Model file for the job. Use its own axes, mm. A direction names the side the tool comes from. Round coordinates to 2 decimals unless told otherwise and drop trailing zeros. Loops run counter-clockwise (first coordinate to the right, second up) from the corner with the lowest first, then second, coordinate; pieces in that order, holes last. Notation, with made-up numbers: (49.25, 85) - (64.25, 85) arc R16 cw to (64.25, 101) - close; hole circle Ø9 at (86, 0.5). An arc over 180 degrees is marked (long way). Use one line per item in the form item = value.
from build123d import *

# Parameters (mm, degrees)
F0_W     = 2032
F0_H     = 508
F1_DEPTH = 762
F2_W     = 591.2553668022
F2_H     = 534.2325568199
F3_DEPTH = 2032


with BuildPart() as f1:
    # F0 (on Front) → F1 (new body)
    with BuildSketch(Plane.XZ):
        Polygon((1016, 0), (0, 0), (-1016, 0), (-1016, -76.2), (1016, -76.2), align=None)
        Polygon((-1016, 0), (0, 0), (1016, 0), (1016, 508), (-1016, 508), align=None)
        with Locations((0, 762)):
            Rectangle(F0_W, F0_H)
        Polygon((-669.1186458851, 1351.5236000156), (-1016, 1016), (1016, 1016), (680.4763999844, 1362.8813541149), align=None)
    extrude(amount=F1_DEPTH)

    # F2 (on face) → F3 (cut)
    with BuildSketch(Plane(origin=(-1016, 0, 0), x_dir=(0, -1, 0), z_dir=(-1, 0, 0))):
        with Locations((401.707559824, 237.3584806919)):
            Rectangle(F2_W, F2_H)
    extrude(amount=-F3_DEPTH, mode=Mode.SUBTRACT)


solid = f1.part
1. Tool access for faces 1 (the flat face through (-14, -106.08, 234)), 2 (the flat face through (-1016, -376, 720)): list every direction of +Z, -Z, +X, -X, +Y, -Y with a clear straight run to the whole face (end or side of a thin tool).
Geometry check:
face_1 = +X, -X
face_2 = +Z, -Z, -X, +Y, -Y
2. Cut at B-B, the plane y = -425. Give the cut face in (x, z).
Geometry check:
outline = (-1016, -76.2) - (1016, -76.2) - (1016, -29.76) - (-1016, -29.76) - close; (-1016, 504.47) - (1016, 504.47) - (1016, 1016) - (680.48, 1362.88) - (-669.12, 1351.52) - (-1016, 1016) - close
3. Pull direction Z, two halves, no side cores. Call faces 3 (the flat face through (-14, -376, -76.2)), 4 (the flat face through (-14, -697.335, 234)), 5 (the flat face through (1016, -376, 705)), 6 (the flat face through (-14, -398, -29.758)): +Z half, -Z half, draft (parallel to the pull), parting line (faces both ways), or undercut.
Geometry check:
face_3 = -Z half
face_4 = undercut
face_5 = draft
face_6 = undercut
4. Wall check: probe 1 along Y at (x, z) = (304, 341.5); probe 2 along Z at (x, y) = (644, -176); probe 3 along Z at (x, y) = (-57.5, -514). Give the ranges that are in metal, low to high.
Geometry check:
probe_1 = -762 to -697.34, -106.08 to 0
probe_2 = -76.2 to -29.76, 504.47 to 1362.57
probe_3 = -76.2 to -29.76, 504.47 to 1356.67
5. Cut at D-D, the plane y = -69. Give the cut face in (x, z).
Geometry check:
outline = (-1016, -76.2) - (1016, -76.2) - (1016, 1016) - (680.48, 1362.88) - (-669.12, 1351.52) - (-1016, 1016) - close
6. Cut at A-A, the plane z = 233. Give the cut face in (x, y), plus the area to 3 significant figures.
Geometry check:
outline = (-1016, -762) - (1016, -762) - (1016, -697.34) - (-1016, -697.34) - close; (-1016, -106.08) - (1016, -106.08) - (1016, 0) - (-1016, 0) - close
area = 347,000 mm^2
7. Cut at C-C, the plane x = 724.5. Give the cut face in (y, z), plus the area to 3 significant figures.
Geometry check:
outline = (-762, -76.2) - (0, -76.2) - (0, 1317.37) - (-762, 1317.37) - close; hole (-697.34, -29.76) - (-106.08, -29.76) - (-106.08, 504.47) - (-697.34, 504.47) - close
area = 746,000 mm^2
8. Flat gauge pins, fed straight in: pin 1 (1 mm diameter, centred on x = -770, y = -187.5, fed in from +Z); pin 2 (4 mm diameter, centred on x = 307.5, y = -300.5, fed in from +Z). Where does each tip first touch, or does it go through?
Geometry check:
pin_1 = 1254.43
pin_2 = 1359.76
